CAD build for the part. Positions are in the model's coordinates, mm. Give positions to 0.01 mm unless a question says otherwise; leave off trailing zeros. Loops run counter-clockwise (first coordinate to the right, second up) from the corner with the lowest first, then second, coordinate; pieces in that order, holes last. Notation, with made-up numbers: (49, 82.5) - (70, 82.5) arc R22 ccw to (70, 108.5) - close; hole circle Ø8 at (-23.5, 76.5). An arc over 180 degrees is marked (long way). Return JSON: item names as keys, results as strings.
from build123d import *

# Parameters (mm, degrees)
PAD_DEPTH = 3


with BuildPart() as part:
    # Sketch (on XY_Plane of Origin) → Pad (new body)
    with BuildSketch(Plane.XY):
        with BuildLine():
            Line((6.28, 0), (247.72, 0))
            ThreePointArc((247.72, 0), (252.160631, 1.839369), (254, 6.28))
            Line((254, 6.28), (254, 38.12))
            ThreePointArc((254, 38.12), (252.160631, 42.560631), (247.72, 44.4))
            Line((247.72, 44.4), (6.28, 44.4))
            ThreePointArc((6.28, 44.4), (1.839369, 42.560631), (0, 38.12))
            Line((0, 38.12), (0, 6.28))
            ThreePointArc((0, 6.28), (1.839369, 1.839369), (6.28, 0))
        make_face()
        with BuildLine():
            ThreePointArc((243.765, 9.575), (240.515, 6.325), (243.765, 3.075))
            Line((243.765, 3.075), (246.765, 3.075))
            ThreePointArc((246.765, 3.075), (250.015, 6.325), (246.765, 9.575))
            Line((243.765, 9.575), (246.765, 9.575))
        make_face(mode=Mode.SUBTRACT)
        with BuildLine():
            ThreePointArc((243.765, 41.325), (240.515, 38.075), (243.765, 34.825))
            Line((243.765, 34.825), (246.765, 34.825))
            ThreePointArc((246.765, 34.825), (250.015, 38.075), (246.765, 41.325))
            Line((243.765, 41.325), (246.765, 41.325))
        make_face(mode=Mode.SUBTRACT)
        with BuildLine():
            ThreePointArc((7.235, 9.575), (3.985, 6.325), (7.235, 3.075))
            Line((7.235, 3.075), (10.235, 3.075))
            ThreePointArc((10.235, 3.075), (13.485, 6.325), (10.235, 9.575))
            Line((7.235, 9.575), (10.235, 9.575))
        make_face(mode=Mode.SUBTRACT)
        with BuildLine():
            ThreePointArc((7.235, 41.325), (3.985, 38.075), (7.235, 34.825))
            Line((7.235, 34.825), (10.235, 34.825))
            ThreePointArc((10.235, 34.825), (13.485, 38.075), (10.235, 41.325))
            Line((7.235, 41.325), (10.235, 41.325))
        make_face(mode=Mode.SUBTRACT)
    extrude(amount=PAD_DEPTH)


solid = part.part
1. Cut at A-A, the plane z = 1.7. Write the cut outline in (x, y) (3 decimals).
Values follow:
{"outline": "(0, 6.28) arc R6.28 ccw to (6.28, 0) - (247.72, 0) arc R6.28 ccw to (254, 6.28) - (254, 38.12) arc R6.28 ccw to (247.72, 44.4) - (6.28, 44.4) arc R6.28 ccw to (0, 38.12) - close; hole (7.235, 3.075) - (10.235, 3.075) arc R3.25 ccw to (10.235, 9.575) - (7.235, 9.575) arc R3.25 ccw to start; hole (7.235, 34.825) - (10.235, 34.825) arc R3.25 ccw to (10.235, 41.325) - (7.235, 41.325) arc R3.25 ccw to start; hole (243.765, 3.075) - (246.765, 3.075) arc R3.25 ccw to (246.765, 9.575) - (243.765, 9.575) arc R3.25 ccw to start; hole (243.765, 34.825) - (246.765, 34.825) arc R3.25 ccw to (246.765, 41.325) - (243.765, 41.325) arc R3.25 ccw to start"}
2. Drill centre lines: probe 1 along X at (y, z) = (6, 1.25); probe 2 along X at (y, z) = (40, 2.2); probe 3 along X at (y, z) = (2, 2.3). Where is each one in solid material? Low to high.
Values follow:
{"probe 1": "x = 0.01 to 4, 13.47 to 240.53, 250 to 253.99", "probe 2": "x = 0.29 to 4.62, 12.85 to 241.15, 249.38 to 253.71", "probe 3": "x = 1.68 to 252.32"}
3. Pull direction Z, two halves, no side cores. Call faces 1 (the face through (125, 23, 0)), 2 (the face through (125, 23, 3)), 3 (the face through (1.89, 42.61, 1.48)): +Z half, -Z half, draft (parallel to the pull), parting line (faces both ways), or undercut.
Values follow:
{"face 1": "-Z half", "face 2": "+Z half", "face 3": "draft"}
4. Drop a flat-ended pin along its axis: P1, Ø2, axis at x = 157, y = 9.5, coming from the -Z side. Give the stop position or say it passes through.
Values follow:
{"P1": "stops at z = 0"}
